For this review, take the finished solid that the model builds, in its own axes (mm). A direction names the side the tool comes from. Coordinates: 2 decimals unless noted, no trailing zeros. Write each loop counter-clockwise with the first axis right and the second up, starting at its lowest first coordinate (ties: lowest second). Pieces come first, ordered by that corner, then holes. Notation, with made-up numbers: M 71,49 L 81,49 A32 ccw 81,78 Z; hole C 42,60.25 d7. An arc over 180 degrees is marked long. Return JSON: item names as keys, results as strings.
```python
from build123d import *

# Parameters (mm, degrees)
F1_DEPTH       = 5
F4_D           = 3.1
F4_CSINK_D     = 6
F4_CSINK_ANGLE = 90
F5_D           = 3.1
F5_CSINK_D     = 6
F5_CSINK_ANGLE = 90
F6_R           = 5
F7_R           = 5


with BuildPart() as f1:
    # F0 (on Top) → F1 (new body, symmetric)
    with BuildSketch(Plane.XY):
        Polygon((-37.666672, 6.7), (-37.666672, 0), (-17.666672, 0), (-17.666672, 20.000001), (-24.366672, 20), (-24.366672, 6.7), align=None)
    extrude(amount=F1_DEPTH, both=True)

    # F4 (through all)
    with Locations(Plane(origin=(-24.366672, 0, 0), x_dir=(0, -1, 0), z_dir=(-1, 0, 0))):
        with Locations((-11.7, 0)):
            CounterSinkHole(F4_D / 2, F4_CSINK_D / 2, counter_sink_angle=F4_CSINK_ANGLE)

    # F5 (through all)
    with Locations(Plane(origin=(0, 6.7, 0), x_dir=(-1, 0, 0), z_dir=(0, 1, 0))):
        with Locations((29.366672, 0)):
            CounterSinkHole(F5_D / 2, F5_CSINK_D / 2, counter_sink_angle=F5_CSINK_ANGLE)

    # F6
    f6_edges = [f1.edges().sort_by_distance(p)[0] for p in [
        (-17.666672, 0, 0),
    ]]
    fillet(f6_edges, radius=F6_R)

    # F7
    f7_edges = [f1.edges().sort_by_distance(p)[0] for p in [
        (-24.366672, 20, 0),
        (-37.666672, 6.7, 0),
    ]]
    fillet(f7_edges, radius=F7_R)


solid = f1.part
```
1. We need section A-A (z = 0). State the section outline as (x, y) points.
Checks:
{"outline": "M -37.67,0 L -30.92,0 L -30.92,5.25 L -32.37,6.7 L -32.67,6.7 A5 ccw -37.67,1.7 Z; M -27.82,0 L -22.67,0 A5 ccw -17.67,5 L -17.67,10.15 L -22.92,10.15 L -24.37,8.7 L -24.37,6.7 L -26.37,6.7 L -27.82,5.25 Z; M -24.37,14.7 L -22.92,13.25 L -17.67,13.25 L -17.67,20 L -19.37,20 A5 ccw -24.37,15 Z"}
2. For faces 5 (the face through (-19, 20, 0)), 6 (the face through (-24.367, 8, 0)), list the 3-axis set-ups (+Z, -Z, +X, -X, +Y, -Y) from which the entire face can be reached by the end or side of a thin tool; tool diameter is ignored.
Checks:
{"face 5": "+Z, -Z, +X, -X, +Y", "face 6": "+Z, -Z, -X, +Y"}
3. We need section B-B (y = 11.7). State the section outline as (x, z) points, plus the area to 3 significant figures.
Checks:
{"outline": "M -24.37,-5 L -17.67,-5 L -17.67,-1.55 L -22.92,-1.55 L -24.37,-3 Z; M -24.37,3 L -22.92,1.55 L -17.67,1.55 L -17.67,5 L -24.37,5 Z", "area": "44.1 mm2"}
4. We need section D-D (y = 18). State the section outline as (x, z) points, plus the area to 3 significant figures.
Checks:
{"outline": "M -23.37,-5 L -17.67,-5 L -17.67,5 L -23.37,5 Z", "area": "57.0 mm2"}
5. Draft analysis for pull direction Y (two halves, no side actions). For faces 1 (the face through (-23, 8, 5)), 2 (the face through (-20.255, 13.178, 0.466)), 3 (the face through (-36.24, 5.2, -0.07)), 4 (the face through (-19.092, 1.504, 0.07)), state which applies: +Y half, -Y half, draft (parallel to the pull), parting line (faces both ways), or undercut.
Checks:
{"face 1": "draft", "face 2": "undercut", "face 3": "+Y half", "face 4": "-Y half"}
6. Wall thickness on L1, parallel to X at y = 7.5, z = 4; L2, parallel to Y at x = -24.5, z = 0; L3, parallel to Y at x = -19.25, z = 0: over which ranges is each line inside the solid? List them lowest first. Write a range as from..to.
Checks:
{"L1": "-24.37..-17.67", "L2": "0..6.7", "L3": "1.35..10.15, 13.25..20"}
7. We need section C-C (x = -20.75). State the section outline as (y, z) points, plus the area to 3 significant figures.
Checks:
{"outline": "M 0.38,-5 L 19.8,-5 L 19.8,5 L 0.38,5 Z; hole C 11.7,0 d3.1", "area": "187 mm2"}
8. Clearance check with flat-ended pins moving along their axes: pin 1 Ø4 at (x, z) = (-23.5, 4) entering from +Y; pin 2 Ø4 at (x, z) = (-29, 0) entering from +Y; pin 3 Ø2 at (x, z) = (-35, 3.5) entering from +Y. State where each tip first meets the part, or that it passes through.
Checks:
{"pin 1": "y = 19.52", "pin 2": "y = 6.07", "pin 3": "y = 6.52"}
